Build history of the part. All positions in model axes, mm. Give positions to 0.01 mm unless a question says otherwise; leave off trailing zeros. Order: outer loops, then holes, each group sorted by start corner. A loop starts at its lowest first (then second) coordinate and runs counter-clockwise, first axis right, second up. Notation, with made-up numbers: (51.25, 14) - (97.25, 14) arc R11 ccw to (97.25, 33) - close; hole circle Ø9 at (-19.75, 81). An arc over 180 degrees is marked (long way). One line per item, written item: value.
Autodesk Inventor part; units mm, degrees
ref_plane "Work Plane1" through (7.5, 7.7044, 240) normal (0, 0, 1) x (1, 0, 0)
ref_plane "YZ Plane" through (0, 0, 0) normal (1, 0, 0) x (0, 1, 0)
ref_plane "XZ Plane" through (0, 0, 0) normal (0, 1, 0) x (-1, 0, 0)
sketch "Sketch1" plane through (0, 0, 0) normal (0, 0, 1) x (1, 0, 0)
  line L0 (0, 0) -> (15, 0)
  line L1 (15, 0) -> (15, 15)
  line L2 (15, 15) -> (0, 15)
  line L3 (0, 15) -> (0, 0)
  dimension "d0" = 15
  dimension "d1" = 15
extrude "Extrusion1" add sketch "Sketch1" along normal blind 10
sketch "Sketch2" plane through (0, 0, 10) normal (0, 0, 1) x (1, 0, 0)
  line L0 (15, 15) -> (0, 15)
  line L1 (0, 15) -> (7.5, 15)
  line L2 (7.5, 15) -> (7.5, 0.4087)
  line L3 (0, 15) -> (0, 0)
  line L4 (0, 7.7044) -> (14.7572, 7.5)
  circle A0 centre (7.5, 7.7044) radius 4.5
  dimension "d9" = 9
extrude "Extrusion2" add sketch "Sketch2" along normal blind 230 contours A0 L4 L2 | L2 L4 A0 | L4 A0 L2 | L2 A0 L4
thread "Thread1"
thread "Thread2"
sketch "Sketch3" plane through (0, 0, 0) normal (1, 0, 0) x (0, 1, 0)
  point P0 (0, 0)
ref_plane "Work Plane1" through (7.5, 7.7044, 240) normal (0, 0, 1) x (1, 0, 0)
sketch "Sketch4" plane through (7.5, 7.7044, 240) normal (0, 0, 1) x (1, 0, 0)
  point P0 (-7.5, -7.7044)
extrude "Extrusion3" [suppressed]
properties part number "23CM NUT"
(1) Slice it at A-A, the plane x = 7.5. Give the cut face in (y, z).
Completed:
outline: (0, 0) - (15, 0) - (15, 10) - (12.2, 10) - (12.2, 240) - (3.2, 240) - (3.2, 10) - (0, 10) - close
(2) Drill centre lines: line 1 (Z direction, x = 12.25, y = 8.25); line 2 (X direction, y = 8.25, z = 156); line 3 (Y direction, x = 7.75, z = 108.5). Where is each one in solid material? Low to high.
Completed:
line 1: 0 to 10
line 2: 3.03 to 11.97
line 3: 3.21 to 12.2
(3) Pin check, flat tips, straight feed: P1, Ø8, axis at x = 9.5, z = 94.5, coming from the -Y side; P2, Ø1.5, axis at x = 4.5, z = 111, coming from the -Y side; P3, Ø2, axis at x = 2.5, z = 122.5, coming from the -Y side. Stop position of each tip, or through.
Completed:
P1: y = 3.2
P2: y = 3.81
P3: y = 5.64
(4) Slice it at C-C, the plane z = 100.5. Give the cut face in (x, y), and give its area (3 significant figures).
Completed:
outline: circle Ø9 at (7.5, 7.7)
area: 63.6 mm²
(5) Slice it at B-B, the plane y = 10. Give the cut face in (x, z), and give its area (3 significant figures).
Completed:
outline: (0, 0) - (15, 0) - (15, 10) - (11.37, 10) - (11.37, 240) - (3.63, 240) - (3.63, 10) - (0, 10) - close
area: 1,930 mm²
(6) Pull direction X, two halves, no side cores. Call faces 1 (the face through (4, 4, 10)), 2 (the face through (11.79, 6.35, 123.39)), 3 (the face through (0, 8, 5)): +X half, -X half, draft (parallel to the pull), parting line (faces both ways), or undercut.
Completed:
face 1: draft
face 2: parting line
face 3: -X half
